Autodesk Inventor part; units mm, degrees
ref_plane "YZ Plane" through (0, 0, 0) normal (1, 0, 0) x (0, 1, 0)
ref_plane "XZ Plane" through (0, 0, 0) normal (0, 1, 0) x (-1, 0, 0)
ref_plane "XY Plane" through (0, 0, 0) normal (0, 0, 1) x (1, 0, 0)
sketch "Sketch1" plane through (0, 0, 0) normal (0, 1, 0) x (-1, 0, 0)
  line L0 (24, 24) -> (-24, 24)
  line L1 (-24, 24) -> (-24, -24)
  line L2 (-24, -24) -> (24, -24)
  line L3 (24, -24) -> (24, 24)
  line L4 (24, 24) -> (-24, -24) construction
  line L5 (-24, 24) -> (24, -24) construction
  line L6 (-25, 25) -> (25, 25)
  line L7 (25, 25) -> (25, -25)
  line L8 (25, -25) -> (-25, -25)
  line L9 (-25, -25) -> (-25, 25)
  line L10 (-25, 25) -> (25, -25) construction
  line L11 (25, 25) -> (-25, -25) construction
  point P0 (0, 0)
extrude "Extrusion1" add sketch "Sketch1" along normal blind 5
sketch "Sketch2" plane through (0, 5, 0) normal (0, 1, 0) x (1, 0, 0)
  line L0 (-25, -25) -> (25, -25)
  line L1 (25, 25) -> (-25, 25)
  line L2 (-25, -25) -> (25, -25)
  line L3 (25, -25) -> (25, 25)
  line L4 (25, 25) -> (-25, 25)
  line L5 (-25, 25) -> (-25, -25)
  point P0 (0, 0)
extrude "Extrusion2" add sketch "Sketch2" along normal blind 2
sketch "Sketch3" plane through (0, 5, 0) normal (0, -1, 0) x (1, 0, 0)
  line L0 (24, -24) -> (24, 24)
  line L1 (24, 24) -> (-24, 24)
  line L2 (-24, -24) -> (24, -24)
  line L3 (-24, 24) -> (-24, -24)
  circle A0 centre (0, 0) radius 2.75
  line L4 (2.05, 0.585) -> (2.05, -0.585)
  line L5 (-2.05, -0.585) -> (-2.05, 0.585)
  line L6 (-0.585, 2.05) -> (0.585, 2.05)
  line L7 (0.585, -2.05) -> (-0.585, -2.05)
  line L8 (-2.05, 0.585) -> (-0.585, 0.585)
  line L9 (0.585, 0.585) -> (2.05, 0.585)
  line L10 (-0.585, -2.05) -> (-0.585, -0.585)
  line L11 (-0.585, 0.585) -> (-0.585, 2.05)
  line L12 (2.05, -0.585) -> (0.585, -0.585)
  line L13 (-0.585, -0.585) -> (-2.05, -0.585)
  line L14 (0.585, 2.05) -> (0.585, 0.585)
  line L15 (0.585, -0.585) -> (0.585, -2.05)
extrude "Extrusion3" add sketch "Sketch3" along normal blind 3.9 contours A0
fillet "Fillet1" radius 0.3 4 edges at (0.585, 3.05, 0.585) (0.585, 3.05, -0.585) (-0.585, 3.05, 0.585) (-0.585, 3.05, -0.585)
fillet "Fillet2" radius 1.5 1 edges at (-2.75, 5, 0)
Work out the finished part from the listing and answer in its coordinate system (mm). A direction names the side the tool comes from. Round coordinates to 2 decimals unless told otherwise and drop trailing zeros. Loops run counter-clockwise (first coordinate to the right, second up) from the corner with the lowest first, then second, coordinate; pieces in that order, holes last. Notation, with made-up numbers: (13.25, 11.25) -> (70.25, 11.25) arc R22 ccw to (70.25, 22.25) -> close; hole circle Ø10 at (50, 21). An arc over 180 degrees is marked (long way). Use one line per item in the form item = value.
(1) Find section B-B on x = -21.5. Give the vertices of the cut face in (y, z).
Answer list:
outline = (0, -25) -> (7, -25) -> (7, 25) -> (0, 25) -> (0, 24) -> (5, 24) -> (5, -24) -> (0, -24) -> close
(2) Flat-ended cylindrical pins translate along their axes: P1, Ø4.5, axis at x = 1, z = -1, coming from the -Y side; P2, Ø6, axis at x = 6.5, z = -18.5, coming from the -Y side. Find the tip coordinate at first contact, or state that the pin passes through.
Answer list:
P1 = 1.1
P2 = 5
(3) A tool of negligible diameter and unlimited length cuts with its end or side. For faces 1 (the flat face through (0, 3, 25)), 2 (the flat face through (0, 3, 2.05)), from which of +Z, -Z, +X, -X, +Y, -Y can it reach the whole face along a straight path? Write none if from no direction.
Answer list:
face_1 = +Z, +X, -X, +Y, -Y
face_2 = -Y
(4) Find section C-C on z = 18.5. Give the vertices of the cut face in (x, y), then the cut area to 3 significant figures.
Answer list:
outline = (-25, 0) -> (-24, 0) -> (-24, 5) -> (24, 5) -> (24, 0) -> (25, 0) -> (25, 7) -> (-25, 7) -> close
area = 110 mm2
(5) Straight lines are drawn through the part: line 1 (Z direction, x = -12.5, y = 4.75); line 2 (Y direction, x = 19.5, z = 17.5). For each, find the intervals that lie inside material, in ascending order.
Answer list:
line_1 = -25 to -24, 24 to 25
line_2 = 5 to 7
(6) Find section A-A on y = 2.25. Give the vertices of the cut face in (x, z) (3 decimals), then the cut area to 3 significant figures.
Answer list:
outline = (-25, -25) -> (25, -25) -> (25, 25) -> (-25, 25) -> close; circle Ø5.5 at (0, 0); hole (-24, -24) -> (24, -24) -> (24, 24) -> (-24, 24) -> close; hole (-2.05, -0.585) -> (-0.885, -0.585) arc R0.3 cw to (-0.585, -0.885) -> (-0.585, -2.05) -> (0.585, -2.05) -> (0.585, -0.885) arc R0.3 cw to (0.885, -0.585) -> (2.05, -0.585) -> (2.05, 0.585) -> (0.885, 0.585) arc R0.3 cw to (0.585, 0.885) -> (0.585, 2.05) -> (-0.585, 2.05) -> (-0.585, 0.885) arc R0.3 cw to (-0.885, 0.585) -> (-2.05, 0.585) -> close
area = 211 mm2
(7) Find section D-D on x = 0. Give the vertices of the cut face in (y, z).
Answer list:
outline = (0, -25) -> (7, -25) -> (7, 25) -> (0, 25) -> (0, 24) -> (5, 24) -> (5, 4.25) arc R1.5 cw to (3.5, 2.75) -> (1.1, 2.75) -> (1.1, 2.05) -> (5, 2.05) -> (5, -2.05) -> (1.1, -2.05) -> (1.1, -2.75) -> (3.5, -2.75) arc R1.5 cw to (5, -4.25) -> (5, -24) -> (0, -24) -> close
(8) For a pull along X with two mould halves and no side action, classify faces 3 (the cylindrical face through (-0.596, 2.317, 2.685)), 4 (the flat face through (0, 7, 0)), 5 (the flat face through (25, 3, 0)) as released by +X, released by -X, zero draft, split by the parting line, or undercut.
Answer list:
face_3 = undercut
face_4 = zero draft
face_5 = released by +X
